Design review of the part built by this model. Coordinates are the model's own, in mm. A direction names the side the tool comes from. Coordinates: 2 decimals unless noted, no trailing zeros. Write each loop counter-clockwise with the first axis right and the second up, starting at its lowest first coordinate (ties: lowest second). Pieces come first, ordered by that corner, then holes.
Q1. Machinability: for faces 4 (the cylindrical face through (46.304, -33.858, 10.197)), 5 (the flat face through (-49, 1, 1.588)), which of the approach directions +Z, -Z, +X, -X, +Y, -Y give a long, thin tool a straight path to every point of the face, cutting with its end or side? Answer none if there is none.
Q2. Take a section at C-C (z = 14.5). Give the boundary of the cut face in (x, y) (3 decimals).
Q3. Take a section at D-D (z = 26.5). Give the boundary of the cut face in (x, y).
Q4. Insertion check: pin 1 (6 mm diameter, centred on y = -56, z = 9, fed in from +X); pin 2 (15 mm diameter, centred on x = -42.66, y = 42.66, fed in from +Z); pin 3 (1 mm diameter, centred on x = -13, y = 53, fed in from -Z); pin 4 (22 mm diameter, centred on x = 42.66, y = 42.66, fed in from +Z). Each pin has a flat end and moves straight along its axis. Give the tip position at first contact, or say it passes through.
Q5. For probe 1 along Y at (x, z) = (40, 17); probe 2 along Z at (x, y) = (16.5, 49); probe 3 along X at (y, z) = (14.5, 56), list the stretches that pass through material, from the lowest coordinate up.
Q6. Mouldability with a two-part tool opening along X and no side actions: class faces 1 (the cylindrical face through (-3.417, 26.028, 31.306)), 2 (the cylindrical face through (28.77, 9.06, 48.13)), 3 (the flat face through (-32, 32, 19.05)) as pulls with the +X half, pulls with the -X half, needs draft (parallel to the pull), parting line crosses it, or undercut.
```python
from build123d import *

# Parameters (mm, degrees)
SKETCH1_R                 = 76.2
BOSS_EXTRUDE1_DEPTH       = 19.05
SKETCH2_R                 = 9.525
BOLTHOLE_DEPTH            = 110.433918417
BOLTHOLEPATTERN_COUNT     = 4
SKETCH5_OUTSIDE_W         = 197.674
SKETCH5_OUTSIDE_H         = 197.674
SKETCH5_OUTSIDE_R         = 46.0375
RAISED_FACE_DEPTH         = 1.5875
SKETCH8_R                 = 38.8874
WELD_NECK_120_DRAFT_DEPTH = 44.45
WELD_NECK_120_DRAFT_TAPER = 30
WELD_NECK_END_REACH       = 127.08
SKETCH9_R                 = 30.1625
WELD_NECK_CHAMFER1_SIZE   = 1.783344653
WELD_NECK_CHAMFER1_SIZE2  = 2.3241
SKETCH7_R                 = 26.2509
BORE_DEPTH                = 126.080494083
FILLET2_R                 = 1.5875
FILLET3_R                 = 1.5875


with BuildPart() as part:
    # Sketch1 → Boss-Extrude1 (new body)
    with BuildSketch(Plane.XY):
        with Locations(Location((0, 0, 0), (0, 0, 180))):
            Circle(SKETCH1_R)
    extrude(amount=BOSS_EXTRUDE1_DEPTH)

    # Sketch2 → BoltHole (cut, through all)
    with BuildSketch(Plane.XY):
        with Locations(Location((42.656216575, 42.656216575, 0), (0, 0, 180))):
            Circle(SKETCH2_R)
    bolthole = extrude(amount=BOLTHOLE_DEPTH, mode=Mode.SUBTRACT)

    # BoltHolePattern: BoltHole ×4 about axis
    boltholepattern_axis = Axis((0, 0, 0), (0, 0, 1))
    for i in range(1, BOLTHOLEPATTERN_COUNT):
        add(bolthole.rotate(boltholepattern_axis, i * 360 / BOLTHOLEPATTERN_COUNT), mode=Mode.SUBTRACT)

    # Sketch5 outside → Raised Face (cut)
    with BuildSketch(Plane(origin=(0, 0, 0), x_dir=(-1, 0, 0), z_dir=(0, 0, -1))):
        Rectangle(SKETCH5_OUTSIDE_W, SKETCH5_OUTSIDE_H)
        Circle(SKETCH5_OUTSIDE_R, mode=Mode.SUBTRACT)
    extrude(amount=-RAISED_FACE_DEPTH, mode=Mode.SUBTRACT)

    # Sketch8 → Weld Neck 120 Draft (add)
    with BuildSketch(Plane.XY.offset(19.05)):
        Circle(SKETCH8_R)
    extrude(amount=WELD_NECK_120_DRAFT_DEPTH, taper=WELD_NECK_120_DRAFT_TAPER)

    # Sketch9 → Weld Neck End (add, up to next)
    with BuildSketch(Plane.XY.offset(63.5), mode=Mode.PRIVATE) as weld_neck_end_sk1:
        Circle(SKETCH9_R)
    weld_neck_end_tool1 = extrude(weld_neck_end_sk1.sketch, amount=-WELD_NECK_END_REACH, mode=Mode.PRIVATE) - part.part
    add(weld_neck_end_tool1.solids().sort_by_distance((0, 0, 63.5))[0])

    # Weld Neck Chamfer1
    weld_neck_chamfer1_edges = [part.edges().sort_by_distance(p)[0] for p in [
        (-30.1625, 0, 63.5),
    ]]
    weld_neck_chamfer1_side = [part.faces().sort_by_distance(p)[0] for p in [
        (-30.1625, 0, 48.830985045),
    ]]
    chamfer(weld_neck_chamfer1_edges, length=WELD_NECK_CHAMFER1_SIZE, length2=WELD_NECK_CHAMFER1_SIZE2, reference=weld_neck_chamfer1_side[0])

    # Sketch7 → Bore (cut, through all)
    with BuildSketch(Plane.XY):
        Circle(SKETCH7_R)
    extrude(amount=BORE_DEPTH, mode=Mode.SUBTRACT)

    # Fillet2
    fillet2_edges = [part.edges().sort_by_distance(p)[0] for p in [
        (76.2, 0, 1.5875),
        (76.2, 0, 19.05),
    ]]
    fillet(fillet2_edges, radius=FILLET2_R)

    # Fillet3
    fillet3_edges = [part.edges().sort_by_distance(p)[0] for p in [
        (46.0375, 0, 1.5875),
    ]]
    fillet(fillet3_edges, radius=FILLET3_R - 0.0001)  # a hair under: the kernel refuses the full size


solid = part.part
```
Response:
1. face 4: +Z, -Z
1. face 5: -Z
2. outline: circle Ø152.4 at (0, 0); hole circle Ø19.05 at (-42.656, -42.656); hole circle Ø19.05 at (-42.656, 42.656); hole circle Ø52.502 at (0, 0); hole circle Ø19.05 at (42.656, -42.656); hole circle Ø19.05 at (42.656, 42.656)
3. outline: circle Ø69.17 at (0, 0); hole circle Ø52.5 at (0, 0)
4. pin 1: stops at x = 54.75
4. pin 2: passes through
4. pin 3: stops at z = 1.59
4. pin 4: stops at z = 19.05
5. probe 1: y = -64.86 to -51.8, -33.51 to 33.51, 51.8 to 64.86
5. probe 2: z = 1.59 to 19.05
5. probe 3: x = -26.45 to -21.88, 21.88 to 26.45
6. face 1: undercut
6. face 2: parting line crosses it
6. face 3: needs draft
